Job drawing, mm, ordinate dimensions from the low corner. One solid piece. Coordinates: 2 decimals unless noted, no trailing zeros. Loops run counter-clockwise (first coordinate to the right, second up) from the corner with the lowest first, then second, coordinate; pieces in that order, holes last. Notation, with made-up numbers: M 71.5,56 L 100.5,56 A17 ccw 100.5,81 Z; hole C -23,53.25 d7. An arc over 180 degrees is marked long. Write each question's results on one line, items separated by ' | '. Start each with the question number.
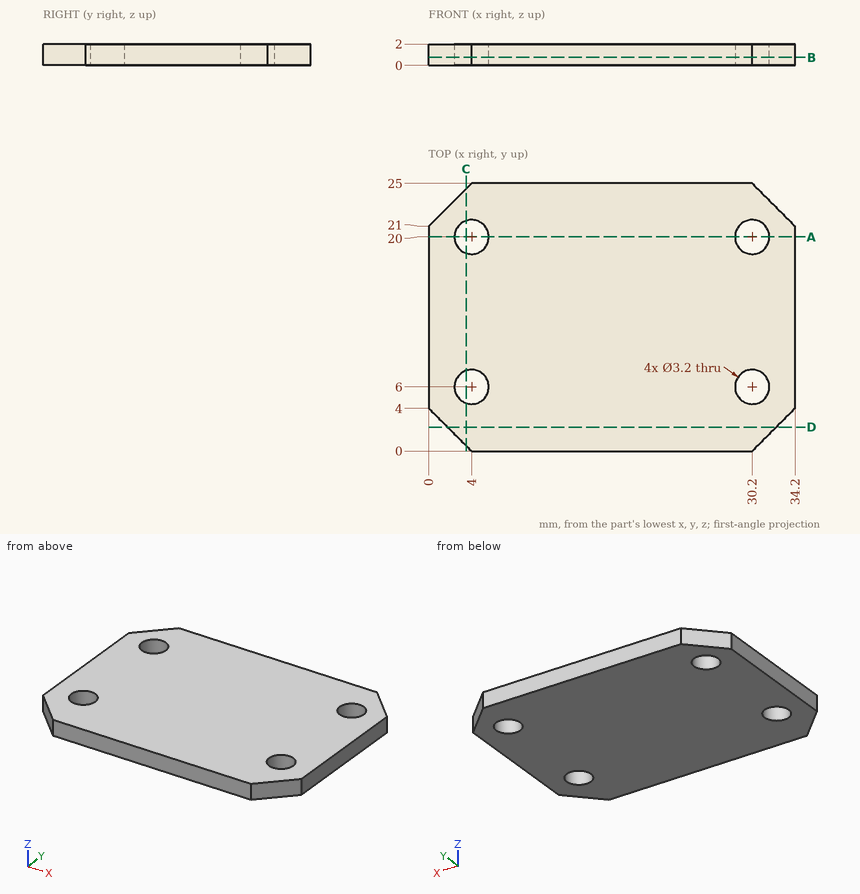
1. Pin check, flat tip, straight feed: pin 1 (1.9 mm diameter, centred on x = 30.2, y = 6, fed in from +Z). Stop position of the tip, or through.
2. Band-saw the part on D-D, the plane y = 2.25. List the corners of the cut face in (x, z), plus the area to 3 significant figures.
3. Band-saw the part on B-B, the plane z = 0.75. List the corners of the cut face in (x, y), plus the area to 3 significant figures.
4. Band-saw the part on A-A, the plane y = 20. List the corners of the cut face in (x, z), plus the area to 3 significant figures.
5. Band-saw the part on C-C, the plane x = 3.5. List the corners of the cut face in (y, z), plus the area to 3 significant figures.
6. Wall check: line 1 along Y through (x, z) = (31.5, 1); line 2 along X through (y, z) = (20.5, 1.85); line 3 along Y through (x, z) = (1, 1.35). Give the ranges that are in metal, low to high.
Checked values:
1) pin 1: through
2) outline: M 1.75,0 L 32.45,0 L 32.45,2 L 1.75,2 Z | area: 61.4 mm²
3) outline: M 0,4 L 4,0 L 30.2,0 L 34.2,4 L 34.2,21 L 30.2,25 L 4,25 L 0,21 Z; hole C 4,6 d3.2; hole C 4,20 d3.2; hole C 30.2,6 d3.2; hole C 30.2,20 d3.2 | area: 791 mm²
4) outline: M 0,0 L 2.4,0 L 2.4,2 L 0,2 Z; M 5.6,0 L 28.6,0 L 28.6,2 L 5.6,2 Z; M 31.8,0 L 34.2,0 L 34.2,2 L 31.8,2 Z | area: 55.6 mm²
5) outline: M 0.5,0 L 4.48,0 L 4.48,2 L 0.5,2 Z; M 7.52,0 L 18.48,0 L 18.48,2 L 7.52,2 Z; M 21.52,0 L 24.5,0 L 24.5,2 L 21.52,2 Z | area: 35.8 mm²
6) line 1: 1.3 to 5.07, 6.93 to 19.07, 20.93 to 23.7 | line 2: 0 to 2.48, 5.52 to 28.68, 31.72 to 34.2 | line 3: 3 to 22
